```python
from build123d import *

# Parameters (mm, degrees)
SKETCH_W   = 210
SKETCH_H   = 125
SKETCH_R   = 6
SKETCH_R_2 = 12
SKETCH_R_3 = 2.5
SKETCH_R_4 = 3.25
SKETCH_R_5 = 1
SKETCH_R_6 = 9.5
SKETCH_R_7 = 3.5
PAD_DEPTH  = 1.5


with BuildPart() as part:
    # Sketch → Pad (new body)
    with BuildSketch(Plane.XY):
        with Locations((105, 62.5)):
            Rectangle(SKETCH_W, SKETCH_H)
        with Locations((15, 108)):
            Circle(SKETCH_R, mode=Mode.SUBTRACT)
        with Locations((15, 86)):
            Circle(SKETCH_R, mode=Mode.SUBTRACT)
        with Locations((15, 64)):
            Circle(SKETCH_R, mode=Mode.SUBTRACT)
        with Locations((15, 42)):
            Circle(SKETCH_R, mode=Mode.SUBTRACT)
        with Locations((15, 20)):
            Circle(SKETCH_R, mode=Mode.SUBTRACT)
        with Locations((176, 101)):
            Circle(SKETCH_R_2, mode=Mode.SUBTRACT)
        with Locations((182, 14)):
            Circle(SKETCH_R_3, mode=Mode.SUBTRACT)
        with Locations((182, 30)):
            Circle(SKETCH_R_3, mode=Mode.SUBTRACT)
        with Locations((160, 30)):
            Circle(SKETCH_R_3, mode=Mode.SUBTRACT)
        with Locations((160, 14)):
            Circle(SKETCH_R_4, mode=Mode.SUBTRACT)
        with Locations((95, 64)):
            Circle(SKETCH_R, mode=Mode.SUBTRACT)
        with Locations((205, 120)):
            Circle(SKETCH_R_5, mode=Mode.SUBTRACT)
        with Locations((37, 108)):
            Circle(SKETCH_R, mode=Mode.SUBTRACT)
        with Locations((37, 86)):
            Circle(SKETCH_R, mode=Mode.SUBTRACT)
        with Locations((37, 64)):
            Circle(SKETCH_R, mode=Mode.SUBTRACT)
        with Locations((37, 42)):
            Circle(SKETCH_R, mode=Mode.SUBTRACT)
        with Locations((37, 20)):
            Circle(SKETCH_R, mode=Mode.SUBTRACT)
        with Locations((59, 108)):
            Circle(SKETCH_R, mode=Mode.SUBTRACT)
        with Locations((59, 86)):
            Circle(SKETCH_R, mode=Mode.SUBTRACT)
        with Locations((59, 64)):
            Circle(SKETCH_R, mode=Mode.SUBTRACT)
        with Locations((59, 42)):
            Circle(SKETCH_R, mode=Mode.SUBTRACT)
        with Locations((59, 20)):
            Circle(SKETCH_R, mode=Mode.SUBTRACT)
        with Locations((95, 20)):
            Circle(SKETCH_R_6, mode=Mode.SUBTRACT)
        with Locations((205, 5)):
            Circle(SKETCH_R_5, mode=Mode.SUBTRACT)
        with Locations((5, 5)):
            Circle(SKETCH_R_5, mode=Mode.SUBTRACT)
        with Locations((5, 120)):
            Circle(SKETCH_R_5, mode=Mode.SUBTRACT)
        with Locations((93, 94)):
            Circle(SKETCH_R_7, mode=Mode.SUBTRACT)
        with Locations((133, 94)):
            Circle(SKETCH_R_7, mode=Mode.SUBTRACT)
    extrude(amount=PAD_DEPTH)


solid = part.part
```
Read the model definition and answer for the solid it produces. Units are mm, in the model's axes. Coordinates: 2 decimals unless noted, no trailing zeros. Loops run counter-clockwise (first coordinate to the right, second up) from the corner with the lowest first, then second, coordinate; pieces in that order, holes last.
(1) The part is cut by section B-B (x = 15). Determine the outline of the cut face in (y, z).
Solution:
outline: (0, 0) - (14, 0) - (14, 1.5) - (0, 1.5) - close; (26, 0) - (36, 0) - (36, 1.5) - (26, 1.5) - close; (48, 0) - (58, 0) - (58, 1.5) - (48, 1.5) - close; (70, 0) - (80, 0) - (80, 1.5) - (70, 1.5) - close; (92, 0) - (102, 0) - (102, 1.5) - (92, 1.5) - close; (114, 0) - (125, 0) - (125, 1.5) - (114, 1.5) - close
(2) The mould has two halves that part along Y. Classify faces 1 (the face through (54.58, 90.06, 0.74)), 2 (the face through (104, 63, 0)): released by +Y, released by -Y, zero draft, split by the parting line, or undercut.
Solution:
face 1: undercut
face 2: zero draft
(3) Flat-ended cylindrical pins translate along their axes: pin 1 Ø9.5 at (x, y) = (37, 108) entering from +Z; pin 2 Ø15.5 at (x, y) = (59, 86) entering from -Z. Find the tip coordinate at first contact, or state that the pin passes through.
Solution:
pin 1: passes through
pin 2: stops at z = 0
(4) Consider line 1 along Y through (x, z) = (133, 1); line 2 along Y through (x, z) = (37, 0.8); line 3 along X through (y, z) = (68.5, 0.7). Determine where each line is inside the solid, lowest interval first.
Solution:
line 1: y = 0 to 90.5, 97.5 to 125
line 2: y = 0 to 14, 26 to 36, 48 to 58, 70 to 80, 92 to 102, 114 to 125
line 3: x = 0 to 11.03, 18.97 to 33.03, 40.97 to 55.03, 62.97 to 91.03, 98.97 to 210
(5) The part is cut by section C-C (z = 0.9). Count the separate pieces of the cut face and the enclosed holes in it, and give its area (3 significant figures).
Solution:
separate pieces: 1
enclosed holes: 28
area: 23,500 mm2
(6) The part is cut by section D-D (x = 160). Determine the outline of the cut face in (y, z).
Solution:
outline: (0, 0) - (10.75, 0) - (10.75, 1.5) - (0, 1.5) - close; (17.25, 0) - (27.5, 0) - (27.5, 1.5) - (17.25, 1.5) - close; (32.5, 0) - (125, 0) - (125, 1.5) - (32.5, 1.5) - close
(7) The part is cut by section A-A (y = 64). Determine the outline of the cut face in (x, z).
Solution:
outline: (0, 0) - (9, 0) - (9, 1.5) - (0, 1.5) - close; (21, 0) - (31, 0) - (31, 1.5) - (21, 1.5) - close; (43, 0) - (53, 0) - (53, 1.5) - (43, 1.5) - close; (65, 0) - (89, 0) - (89, 1.5) - (65, 1.5) - close; (101, 0) - (210, 0) - (210, 1.5) - (101, 1.5) - close
